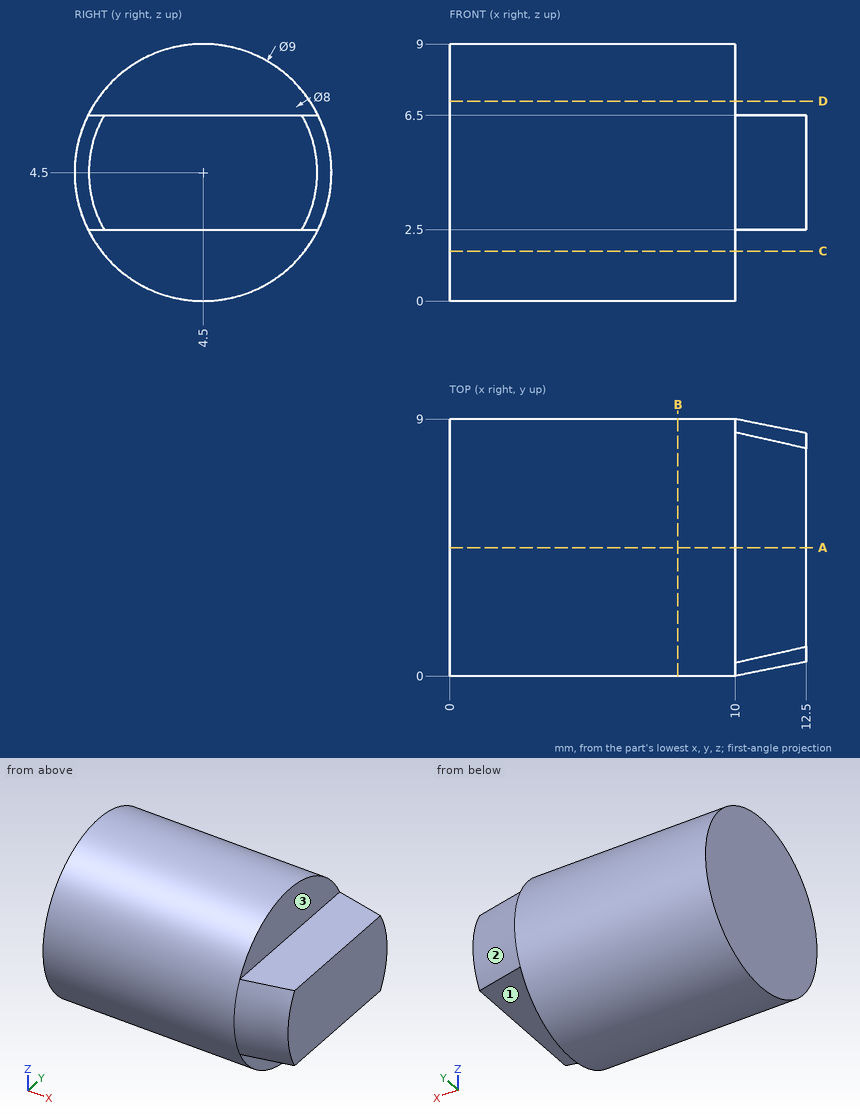
Study the drawing (mm; zero at the part's minimum x, y, z) and answer. A direction names the side the tool comes from. Give positions to 0.01 mm unless a question says otherwise; leave off trailing zeros. Loops run counter-clockwise (first coordinate to the right, second up) from the corner with the lowest first, then second, coordinate; pieces in that order, holes last. Notation, with made-up numbers: M 30,44 L 41,44 A17 ccw 41,49 Z; hole C 26.25,-22.5 d1. An arc over 180 degrees is marked long. Answer as CSV lines item,"result".
Item 1: The part is cut by section C-C (z = 1.75). Give the vertices of the cut face in (x, y).
Values follow:
outline,"M 0,0.94 L 10,0.94 L 10,8.06 L 0,8.06 Z"
Item 2: The part is cut by section A-A (y = 4.5). Give the vertices of the cut face in (x, z).
Values follow:
outline,"M 0,0 L 10,0 L 10,2.5 L 12.5,2.5 L 12.5,6.5 L 10,6.5 L 10,9 L 0,9 Z"
Item 3: Which of the six approach directions +Z, -Z, +X, -X, +Y, -Y give full straight-line access (tool end or side, diameter ignored) to the marked faces 1, 2 and 3?
Values follow:
face 1,"-Z, +X, +Y, -Y"
face 2,"+X, +Y"
face 3,"+Z, +X, +Y, -Y"
Item 4: Given pin 1 Ø0.8 at (y, z) = (5, 1.5) entering from +X; pin 2 Ø1.5 at (y, z) = (7, 5.5) entering from -X; pin 3 Ø1 at (x, y) = (8, 6) entering from -Z; pin 4 Ø3 at (x, y) = (11, 3) entering from -Z, each flat-ended and moving along its own axis, determine where each tip first touches the part or whether it passes through.
Values follow:
pin 1,"stops at x = 10"
pin 2,"stops at x = 0"
pin 3,"stops at z = 0.11"
pin 4,"stops at z = 0.02"
Item 5: Straight lines are drawn through the part: line 1 along X through (y, z) = (6, 6.75); line 2 along Z through (x, y) = (2.75, 2.5); line 3 along Z through (x, y) = (10.25, 8). For each, find the intervals that lie inside material, in ascending order. Write a range as [from, to].
Values follow:
line 1,"x = [0, 10]"
line 2,"z = [0.47, 8.53]"
line 3,"z = [2.5, 6.5]"
Item 6: The part is cut by section D-D (z = 7). Give the vertices of the cut face in (x, y).
Values follow:
outline,"M 0,0.76 L 10,0.76 L 10,8.24 L 0,8.24 Z"
Item 7: The part is cut by section B-B (x = 8). Give the vertices of the cut face in (y, z), and give its area (3 significant figures).
Values follow:
outline,"C 4.5,4.5 d9"
area,"63.6 mm^2"
